Model file for the job. Use its own axes, mm. Face numbers are marked on the shaded views. A direction names the side the tool comes from. Give positions to 0.01 mm unless a question says otherwise; leave off trailing zeros. Write each loop counter-clockwise with the first axis right and the second up, starting at its lowest first coordinate (ties: lowest second). Pieces come first, ordered by that corner, then holes.
```python
from build123d import *

# Parameters (mm, degrees)
SKETCH1_W              = 44
SKETCH1_H              = 360
BASE_FLANGE1_DEPTH     = 1.2
SKETCHED_START         = -22
SKETCHED_BEND1_DEPTH   = 44
SKETCHED_BEND1_2_DEPTH = 44
SKETCH7_R              = 4.5
CUT_EXTRUDE1_DEPTH     = 10
SKETCH8_R              = 4
CUT_EXTRUDE2_DEPTH     = 10


# Read off the part's stored shape, not the designer's step: Sketched Bend1
# Sheet-metal steps are written as plain solids
with BuildPart() as part:
    # Sketch1 → Base-Flange1 (new body)
    with BuildSketch(Plane(origin=(0, 0, 0), x_dir=(1, 0, 0), z_dir=(0, 1, 0))):
        Rectangle(SKETCH1_W, SKETCH1_H)
    extrude(amount=-BASE_FLANGE1_DEPTH)

    # Sketched Bend1 outline → Sketched Bend1 (cut)
    with BuildSketch(Plane.YZ.offset(SKETCHED_START)):
        with BuildLine():
            Line((0, -180), (0, -85.054444388))
            ThreePointArc((0, -85.054444388), (-0.872269031, -84.341342484), (-1.2, -83.2634))
            Line((-1.2, -83.2634), (-1.2, -180))
            Line((-1.2, -180), (0, -180))
        make_face()
    extrude(amount=SKETCHED_BEND1_DEPTH, mode=Mode.SUBTRACT)

    # Sketched Bend1 2 outline → Sketched Bend1 2 (add)
    with BuildSketch(Plane.YZ.offset(SKETCHED_START)):
        with BuildLine():
            Line((93.6, -84), (0.7366, -84))
            ThreePointArc((0.7366, -84), (0.215745145, -83.784254855), (0, -83.2634))
            Line((0, -83.2634), (0, -85.054444388))
            ThreePointArc((0, -85.054444388), (0.361178238, -85.163262642), (0.7366, -85.2))
            Line((0.7366, -85.2), (93.6, -85.2))
            Line((93.6, -85.2), (93.6, -84))
        make_face()
    extrude(amount=SKETCHED_BEND1_2_DEPTH)

    # Sketch7 → Cut-Extrude1 (cut)
    with BuildSketch(Plane(origin=(0, 0, -85.2), x_dir=(-1, 0, 0), z_dir=(0, 0, -1))):
        with Locations(Location((0, 73.6, 0), (0, 0, 90))):
            Circle(SKETCH7_R)
    extrude(amount=-CUT_EXTRUDE1_DEPTH, mode=Mode.SUBTRACT)

    # Sketch8 → Cut-Extrude2 (cut)
    with BuildSketch(Plane.XZ.offset(1.2)):
        with Locations(Location((0, -11.2, 0), (0, 0, 270))):
            Circle(SKETCH8_R)
        with Locations(Location((0, 128.8, 0), (0, 0, 270))):
            Circle(SKETCH8_R)
    extrude(amount=-CUT_EXTRUDE2_DEPTH, mode=Mode.SUBTRACT)


solid = part.part
```
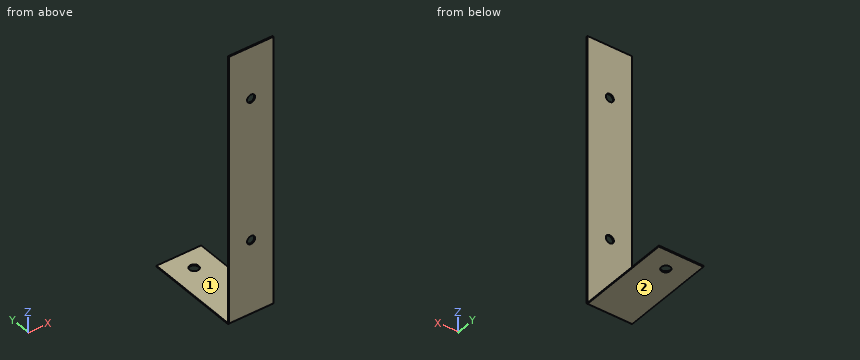
1. Slice it at D-D, the plane z = -66.5. Write the cut outline in (x, y), and give its area (3 significant figures).
Calculated:
outline: (-22, -1.2) - (22, -1.2) - (22, 0) - (-22, 0) - close
area: 52.8 mm2
2. Slice it at A-A, the plane z = -11.2. Write the cut outline in (x, y).
Calculated:
outline: (-22, -1.2) - (-4, -1.2) - (-4, 0) - (-22, 0) - close; (4, -1.2) - (22, -1.2) - (22, 0) - (4, 0) - close
3. Which spindle directions (+Z, -Z, +X, -X, +Y, -Y) get a long thin tool onto all of the face, cutting with end or side? Do the marked faces 1 and 2. Say none if no direction does.
Calculated:
face 1: +Z, +X, -X, +Y
face 2: -Z, +X, -X, +Y, -Y
4. Pin check, flat tips, straight feed: P1, Ø2, axis at x = -13.5, z = 30.5, coming from the +Y side; P2, Ø11.5, axis at x = 0, y = 73.6, coming from the -Z side. Stop position of each tip, or through.
Calculated:
P1: stops at y = 0
P2: stops at z = -85.2
5. Probe probe 1 along X at (y, z) = (-0.7, -11.2); probe 2 along Z at (x, y) = (-11, 55.5); probe 3 along Y at (x, z) = (-17.5, 112.5). List the from-to ranges inside material, lowest first.
Calculated:
probe 1: x = -22 to -4, 4 to 22
probe 2: z = -85.2 to -84
probe 3: y = -1.2 to 0
6. Slice it at B-B, the plane y = 73.6. Write the cut outline in (x, z).
Calculated:
outline: (-22, -85.2) - (-4.5, -85.2) - (-4.5, -84) - (-22, -84) - close; (4.5, -85.2) - (22, -85.2) - (22, -84) - (4.5, -84) - close
7. Slice it at C-C, the plane x = -14. Write the cut outline in (y, z), and give its area (3 significant figures).
Calculated:
outline: (-1.2, -83.26) arc R1.94 ccw to (0.74, -85.2) - (93.6, -85.2) - (93.6, -84) - (0.74, -84) arc R0.74 cw to (0, -83.26) - (0, 180) - (-1.2, 180) - close
area: 430 mm2
